The model under review builds one solid part; all positions refer to its coordinate system, in mm. Face numbers are marked on the shaded views. A direction names the side the tool comes from. Coordinates: 2 decimals unless noted, no trailing zeros. Loops run counter-clockwise (first coordinate to the right, second up) from the corner with the lowest first, then second, coordinate; pieces in that order, holes last. Notation, with made-up numbers: M -28,58.5 L -23,58.5 A20 ccw -23,78.5 Z; hole C 89,27 d1. An arc over 180 degrees is marked long. Return JSON: item names as keys, results as strings.
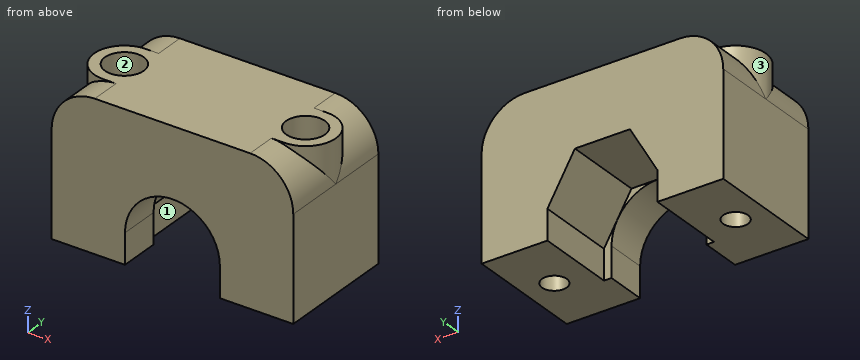
```python
from build123d import *

# Parameters (mm, degrees)
SKETCH1_W           = 56
SKETCH1_H           = 34
BOSS_EXTRUDE1_DEPTH = 28
CUT_EXTRUDE1_DEPTH  = 18.6
CUT_EXTRUDE2_DEPTH  = 9.4
FILLET1_R           = 10
BOSS_EXTRUDE2_DEPTH = 16
SKETCH6_R           = 2.875
CUT_EXTRUDE3_DEPTH  = 34
SKETCH8_R           = 4.5
CUT_EXTRUDE4_DEPTH  = 24


with BuildPart() as part:
    # Sketch1 → Boss-Extrude1 (new body)
    with BuildSketch(Plane(origin=(0, 0, 0), x_dir=(1, 0, 0), z_dir=(0, 1, 0))):
        Rectangle(SKETCH1_W, SKETCH1_H)
    extrude(amount=BOSS_EXTRUDE1_DEPTH)

    # Sketch2 → Cut-Extrude1 (cut)
    with BuildSketch(Plane(origin=(0, 28, 0), x_dir=(1, 0, 0), z_dir=(0, 1, 0))):
        Polygon((-12.75, 10.041823898), (-6.375, -1), (6.375, -1), (12.75, 10.041823898), (12.75, 17), (-12.75, 17), align=None)
    extrude(amount=-CUT_EXTRUDE1_DEPTH, mode=Mode.SUBTRACT)

    # Sketch3 → Cut-Extrude2 (cut)
    with BuildSketch(Plane(origin=(0, 9.4, 0), x_dir=(1, 0, 0), z_dir=(0, 1, 0))):
        with BuildLine():
            Line((-11, 10), (-11, 17))
            Line((-11, 17), (11, 17))
            Line((11, 17), (11, 10))
            ThreePointArc((11, 10), (0, -1), (-11, 10))
        make_face()
    extrude(amount=-CUT_EXTRUDE2_DEPTH, mode=Mode.SUBTRACT)

    # Fillet1
    fillet1_edges = [part.edges().sort_by_distance(p)[0] for p in [
        (28, 14, 17),
        (-28, 14, 17),
    ]]
    fillet(fillet1_edges, radius=FILLET1_R)

    # Sketch5 → Boss-Extrude2 (add)
    with BuildSketch(Plane(origin=(0, 0, 1), x_dir=(-1, 0, 0), z_dir=(0, 0, -1))):
        with BuildLine():
            Line((18, 21), (18, 7))
            Line((18, 7), (21, 7))
            ThreePointArc((21, 7), (28, 14), (21, 21))
            Line((21, 21), (18, 21))
        make_face()
        with BuildLine():
            Line((-18, 7), (-21, 7))
            ThreePointArc((-21, 7), (-28, 14), (-21, 21))
            Line((-21, 21), (-18, 21))
            Line((-18, 21), (-18, 7))
        make_face()
    extrude(amount=-BOSS_EXTRUDE2_DEPTH)

    # Sketch6 → Cut-Extrude3 (cut)
    with BuildSketch(Plane.XY.offset(17)):
        with Locations((-21, 14)):
            Circle(SKETCH6_R)
        with Locations((21, 14)):
            Circle(SKETCH6_R)
    extrude(amount=-CUT_EXTRUDE3_DEPTH, mode=Mode.SUBTRACT)

    # Sketch8 → Cut-Extrude4 (cut)
    with BuildSketch(Plane(origin=(0, 0, -7), x_dir=(-1, 0, 0), z_dir=(0, 0, -1))):
        with Locations((21, 14)):
            Circle(SKETCH8_R)
        with Locations((-21, 14)):
            Circle(SKETCH8_R)
    extrude(amount=-CUT_EXTRUDE4_DEPTH, mode=Mode.SUBTRACT)


solid = part.part
```
1. Add section C-C on z = 2. Give the boundary of the cut face in (x, y), plus the area to 3 significant figures.
Check values:
{"outline": "M -28,0 L 28,0 L 28,28 L -28,28 Z; hole C -21,14 d9; hole C 21,14 d9", "area": "1,440 mm²"}
2. Insertion check: pin 1 Ø8 at (x, y) = (-21, 14) entering from +Z; pin 2 Ø1 at (x, z) = (-10, -6.5) entering from +Y; pin 3 Ø14 at (x, y) = (0.5, 17) entering from -Z. Each pin has a flat end and moves straight along its axis. Give the tip position at first contact, or say it passes through.
Check values:
{"pin 1": "z = -7", "pin 2": "y = 9.4", "pin 3": "z = -0.95"}
3. Add section A-A on z = -2. Give the boundary of the cut face in (x, y).
Check values:
{"outline": "M -28,0 L -7.55,0 L -7.55,9.4 L -8.11,9.4 L -8.11,28 L -28,28 Z; M 7.55,0 L 28,0 L 28,28 L 8.11,28 L 8.11,9.4 L 7.55,9.4 Z; hole C -21,14 d9; hole C 21,14 d9"}
4. To check wall thickness, follow line 1 (Y direction, x = 21, z = 8); line 2 (Z direction, x = 2, y = 16); line 3 (X direction, y = 16, z = 9). State the ranges of each line that lie inside material, in increasing order.
Check values:
{"line 1": "0 to 9.5, 18.5 to 28", "line 2": "1 to 17", "line 3": "-27.8 to -25.03, -16.97 to 16.97, 25.03 to 27.8"}
5. Add section D-D on y = 12.5. State how many separate pieces and enclosed holes the cut face has, plus the area to 3 significant figures.
Check values:
{"separate pieces": "3", "enclosed holes": "0", "area": "1,010 mm²"}
6. Add section B-B on x = -22. Give the boundary of the cut face in (y, z), plus the area to 3 significant figures.
Check values:
{"outline": "M 0,-17 L 11.3,-17 L 11.3,-7 L 9.61,-7 L 9.61,17 L 7.07,17 L 7.07,16.17 L 0,16.17 Z; M 16.7,-17 L 28,-17 L 28,16.17 L 20.93,16.17 L 20.93,17 L 18.39,17 L 18.39,-7 L 16.7,-7 Z", "area": "676 mm²"}
7. Machinability: for the marked faces 1, 2 and 3, which of the approach directions +Z, -Z, +X, -X, +Y, -Y give a long, thin tool a straight path to every point of the face, cutting with its end or side? Answer none if there is none.
Check values:
{"face 1": "-Z, +Y", "face 2": "+Z", "face 3": "+Z, -X"}
